Build history of the part. All positions in model axes, mm. A direction names the side the tool comes from. Round coordinates to 2 decimals unless told otherwise and drop trailing zeros. Loops run counter-clockwise (first coordinate to the right, second up) from the corner with the lowest first, then second, coordinate; pieces in that order, holes last. Notation, with made-up numbers: (46, -40) -> (90, -40) arc R31 cw to (90, -8) -> close; hole circle Ø9 at (-13, 64). An arc over 180 degrees is marked (long way). Put each result on its own line as item: value. Start each with the question number.
Item 1: Flat gauge pins, fed straight in: pin 1 Ø1.7 at (y, z) = (1, 2.5) entering from -X; pin 2 Ø0.8 at (y, z) = (4.5, 7) entering from +X; pin 3 Ø8 at (y, z) = (8, 6) entering from +X. Where does each tip first touch, or does it go through?
Item 2: Drill centre lines: probe 1 along X at (y, z) = (-19, 15); probe 2 along Z at (x, y) = (117.5, 9); probe 3 along Y at (x, z) = (-45, 12.5). Where is each one in solid material? Low to high. Write a range as [from, to].
Item 3: Pull direction Z, two halves, no side cores. Call faces 1 (the flat face through (27, 0, 28)), 2 (the flat face through (19, -5, 17.78)), 3 (the flat face through (106, -4, 17.78)): +Z half, -Z half, draft (parallel to the pull), parting line (faces both ways), or undercut.
Item 4: Tool access for faces 4 (the flat face through (19, -10.16, 20)), 5 (the flat face through (-6, -3, 7.112)), 6 (the flat face through (-80, 4, 7.62)), 7 (the flat face through (-13, -5.08, 4)), 8 (the flat face through (-6, 3, 6.35)): list every direction of +Z, -Z, +X, -X, +Y, -Y with a clear straight run to the whole face (end or side of a thin tool).
Item 5: Cut at D-D, the plane z = 43. List the corners of the cut face in (x, y), plus the area to 3 significant figures.
Item 6: Cut at A-A, the plane y = -16. List the corners of the cut face in (x, z), plus the area to 3 significant figures.
Item 7: Cut at B-B, the plane y = 4. Count the separate pieces of the cut face and the enclosed holes in it, plus the area to 3 significant figures.
Item 8: Cut at C-C, the plane x = 61. List the corners of the cut face in (y, z), plus the area to 3 significant figures.
```python
from build123d import *

# Parameters (mm, degrees)
F2_W      = 76.2
F2_H      = 5.08
F3_DEPTH  = 9.398
F5_W      = 38.1
F5_H      = 10.16
F5_W_2    = 4.6505859673
F5_H_2    = 5.3134663665
F11_DEPTH = 4.572
F7_W      = 10.16
F7_H      = 10.16
F7_R      = 1.27
F7_W_2    = 63.5
F12_DEPTH = 10.16
F8_R      = 1.27
F2_R      = 1.27
F0_W      = 12.7
F0_H      = 5.08
F19_DEPTH = 7.62
F20_DEPTH = 7.112
F0_W_2    = 6.35
F0_H_2    = 1.524
F21_DEPTH = 6.35
F22_DEPTH = 7.62
F17_W     = 0.508
F17_H     = 1.524
F17_H_2   = 1.27
F23_DEPTH = 2.54
F24_W     = 86.36
F24_H     = 86.36
F25_DEPTH = 30.48
F26_W     = 55.88
F26_H     = 55.88
F27_DEPTH = 7.62
F28_DEPTH = 5.08


with BuildPart() as f3:
    # F2 (on offset) → F3 (new body)
    with BuildSketch(Plane.XY.offset(7.62)):
        with Locations((-20.32, 4.064)):
            Rectangle(F2_W, F2_H)
        Polygon((17.78, 0), (0, 0), (0, -5.08), (0, -10.16), (17.78, -10.16), (17.78, -5.08), align=None)
        with BuildLine():
            Line((17.78, 1.524), (17.78, 0))
            Line((17.78, 0), (17.78, -5.08))
            Line((17.78, -5.08), (17.78, -10.16))
            ThreePointArc((17.78, -10.16), (26.162, -1.778), (17.78, 6.604))
            Line((17.78, 6.604), (17.78, 1.524))
        make_face()
    extrude(amount=F3_DEPTH)



with BuildPart() as f11:
    # F5 (on offset) → F11 (new body)
    with BuildSketch(Plane.XY.offset(17.78)):
        with Locations((19.05, -5.08)):
            Rectangle(F5_W, F5_H)
        with Locations((25.4, -5.08)):
            Rectangle(F5_W_2, F5_H_2, mode=Mode.SUBTRACT)
    extrude(amount=F11_DEPTH)

    # F15: sweep along a path in F14
    with BuildLine(Plane.XZ.offset(1.905)) as f15_path:
        Line((0, 20.32), (-22.86, 20.32))
        Line((-22.86, 20.32), (-22.86, 7.62))
    # F8 (on Right) + F2 (on offset) → F15 (sweep)
    with BuildSketch(Plane.YZ):
        with Locations((-1.905, 20.32)):
            Circle(F8_R)
    with BuildSketch(Plane.XY.offset(7.62)):
        with Locations((-22.86, -1.905)):
            Circle(F2_R)
    sweep(path=f15_path.line, transition=Transition.RIGHT)


with BuildPart() as f12:
    # F7 (on offset) → F12 (new body)
    with BuildSketch(Plane.XY.offset(22.86)):
        with Locations((-5.08, -5.08)):
            Rectangle(F7_W, F7_H)
        with Locations((-5.08, -8.255)):
            Circle(F7_R, mode=Mode.SUBTRACT)
        with Locations((31.75, -5.08)):
            Rectangle(F7_W_2, F7_H)
        with Locations((-5.08, -8.255)):
            Circle(F7_R)
    extrude(amount=F12_DEPTH)


with BuildPart() as f3_1:
    add(f3.part)

    add(f12.part)  # F18 merges F12
    # F18: sweep along a path in F10
    with BuildLine(Plane.XZ.offset(8.255)) as f18_path:
        Line((-5.08, 22.86), (-5.08, 13.335))
        Line((-5.08, 13.335), (0, 13.335))
    # F8 (on Right) + F7 (on offset) → F18 (sweep)
    with BuildSketch(Plane.YZ):
        with Locations((-8.3337165415, 13.335)):
            Circle(F8_R)
    with BuildSketch(Plane.XY.offset(22.86)):
        with Locations((-5.08, -8.255)):
            Circle(F7_R)
    sweep(path=f18_path.line, transition=Transition.RIGHT)

    # F24 (on offset) → F25 (join)
    with BuildSketch(Plane.XY.offset(17.78)):
        with Locations((106.68, -5.08)):
            Rectangle(F24_W, F24_H)
    extrude(amount=F25_DEPTH)


    add(f11.part)  # F27 merges F11


with BuildPart() as f19:
    # F0 (on Top) → F19 (new body)
    with BuildSketch(Plane.XY):
        with Locations((-19.05, -2.54)):
            Rectangle(F0_W, F0_H)
    extrude(amount=F19_DEPTH)

    # F0 (on Top) → F20 (join)
    with BuildSketch(Plane.XY):
        Polygon((0, -5.08), (0, 0), (-6.35, 0), (-12.7, 0), (-12.7, -5.08), align=None)
    extrude(amount=F20_DEPTH)

    # F0 (on Top) → F21 (join)
    with BuildSketch(Plane.XY):
        with Locations((-3.175, 0.762)):
            Rectangle(F0_W_2, F0_H_2)
        Polygon((-6.35, 1.524), (0, 1.524), (0, 6.604), (-12.7, 6.604), (-12.7, 1.524), align=None)
    extrude(amount=F21_DEPTH)


with BuildPart() as f22:
    # F0 (on Top) → F22 (new body)
    with BuildSketch(Plane.XY):
        with Locations((-19.05, 4.064)):
            Rectangle(F0_W, F0_H)
    extrude(amount=F22_DEPTH)

    # F17 (on offset) → F23 (cut, symmetric)
    with BuildSketch(Plane.XZ.offset(-4.064)):
        with Locations((-12.954, 5.842)):
            Rectangle(F17_W, F17_H)
        with Locations((-25.146, 0.635)):
            Rectangle(F17_W, F17_H_2)
        with Locations((-19.05, 3.175)):
            Rectangle(F17_W, F17_H_2)
        with Locations((-16.002, 4.445)):
            Rectangle(F17_W, F17_H_2)
        with Locations((-22.098, 1.905)):
            Rectangle(F17_W, F17_H_2)
    extrude(amount=F23_DEPTH, both=True, mode=Mode.SUBTRACT)


with BuildPart() as f3_2:
    add(f3_1.part)

    add(f19.part)  # F27 merges F19

    add(f22.part)  # F27 merges F22
    # F26 (on offset) → F27 (join)
    with BuildSketch(Plane.XY.offset(7.62)):
        with Locations((-86.36, 4.064)):
            Rectangle(F26_W, F26_H)
    extrude(amount=F27_DEPTH)

    # F5 (on offset) → F28 (join)
    with BuildSketch(Plane.XY.offset(17.78)):
        with Locations((25.4, -5.08)):
            Rectangle(F5_W_2, F5_H_2)
    extrude(amount=F28_DEPTH)


solid = f3_2.part
```
Reply:
1. pin 1: stops at x = -25.4
1. pin 2: stops at x = -12.7
1. pin 3: stops at x = 23.51
2. probe 1: x = [-114.3, -58.42]
2. probe 2: z = [17.78, 48.26]
2. probe 3: y = [1.52, 6.6]
3. face 1: draft
3. face 2: undercut
3. face 3: -Z half
4. face 4: +Z, -Z, -X, -Y
4. face 5: +X, +Y, -Y
4. face 6: -Z, -X, +Y, -Y
4. face 7: -Z, +X, -X, -Y
4. face 8: +X, +Y
5. outline: (63.5, -48.26) -> (149.86, -48.26) -> (149.86, 38.1) -> (63.5, 38.1) -> close
5. area: 7,460 mm^2
6. outline: (-114.3, 7.62) -> (-58.42, 7.62) -> (-58.42, 15.24) -> (-114.3, 15.24) -> close; (63.5, 17.78) -> (149.86, 17.78) -> (149.86, 48.26) -> (63.5, 48.26) -> close
6. area: 3,060 mm^2
7. separate pieces: 2
7. enclosed holes: 3
7. area: 4,010 mm^2
8. outline: (-10.16, 22.86) -> (0, 22.86) -> (0, 33.02) -> (-10.16, 33.02) -> close
8. area: 103 mm^2
